```python
from build123d import *

# Parameters (mm, degrees)
SKETCH1_W           = 762
SKETCH1_H           = 101.6
SKETCH1_W_2         = 76.2
SKETCH1_H_2         = 558.8
BOSS_EXTRUDE1_DEPTH = 215.9
SKETCH2_R           = 6.35
CUT_EXTRUDE1_DEPTH  = 432.8


with BuildPart() as part:
    # Sketch1 → Boss-Extrude1 (new body, symmetric)
    with BuildSketch(Plane.XY):
        Rectangle(SKETCH1_W, SKETCH1_H)
        with Locations((190.5, 330.2)):
            Rectangle(SKETCH1_W_2, SKETCH1_H_2)
    extrude(amount=BOSS_EXTRUDE1_DEPTH, both=True)

    # Sketch2 → Cut-Extrude1 (cut, through all)
    with BuildSketch(Plane.XY.offset(215.9)):
        with Locations((190.5, 590.55)):
            Circle(SKETCH2_R)
    extrude(amount=-CUT_EXTRUDE1_DEPTH, mode=Mode.SUBTRACT)


solid = part.part
```
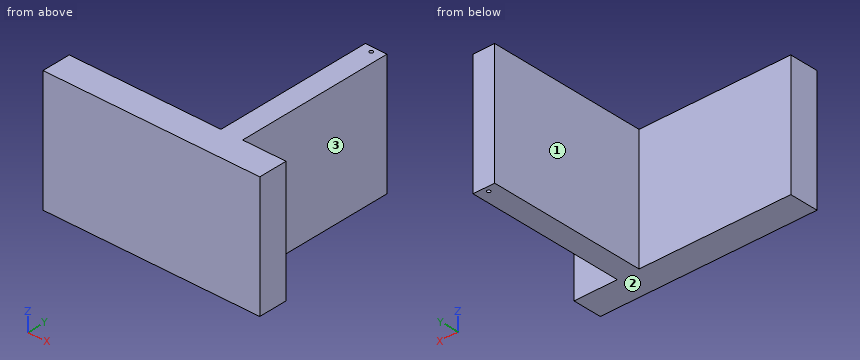
Could you check a few things on this model? Use its own coordinates, in mm. Face numbers are marked on the shaded views. A direction names the side the tool comes from. Round coordinates to 2 decimals unless told otherwise and drop trailing zeros. Loops run counter-clockwise (first coordinate to the right, second up) from the corner with the lowest first, then second, coordinate; pieces in that order, holes last.
Q1. For P1, Ø1, axis at x = -66, z = -92, coming from the +Y side; P2, Ø12, axis at y = 425, z = 111, coming from the -X side; P3, Ø11.5, axis at x = 190.5, y = 590.55, coming from the -Z side; P4, Ø5, axis at y = 120, z = 138.5, coming from the +X side, each with a flat end and sliding along its axis, tell me the tip position at first contact or that it passes through.
Q2. I want a section at B-B (x = 51.5). Write out the boundary of the cut face in (y, z).
Q3. Please list where these lines run through material, in increasing order: L1, parallel to X at y = 590.55, z = -115; L2, parallel to Y at x = 190, z = 34; L3, parallel to Y at x = 291, z = -172.5.
Q4. I want a section at C-C (y = 478). Write out the boundary of the cut face in (x, z).
Q5. On a 3-axis mill with a long thin cutter (end or side, diameter ignored), from which of +Z, -Z, +X, -X, +Y, -Y can I reach the whole of each face in a straight line? I mean the marked faces 1, 2 and 3. Say none if no direction works.
Q6. I want a section at A-A (z = 95). Write out the boundary of the cut face in (x, y).
Answer below:
1. P1: stops at y = 50.8
1. P2: stops at x = 152.4
1. P3: passes through
1. P4: stops at x = 228.6
2. outline: (-50.8, -215.9) - (50.8, -215.9) - (50.8, 215.9) - (-50.8, 215.9) - close
3. L1: x = 152.4 to 184.15, 196.85 to 228.6
3. L2: y = -50.8 to 584.22, 596.88 to 609.6
3. L3: y = -50.8 to 50.8
4. outline: (152.4, -215.9) - (228.6, -215.9) - (228.6, 215.9) - (152.4, 215.9) - close
5. face 1: +Z, -Z, -X, +Y
5. face 2: -Z, +X, -X, +Y, -Y
5. face 3: +Z, -Z, +X, +Y
6. outline: (-381, -50.8) - (381, -50.8) - (381, 50.8) - (228.6, 50.8) - (228.6, 609.6) - (152.4, 609.6) - (152.4, 50.8) - (-381, 50.8) - close; hole circle Ø12.7 at (190.5, 590.55)
